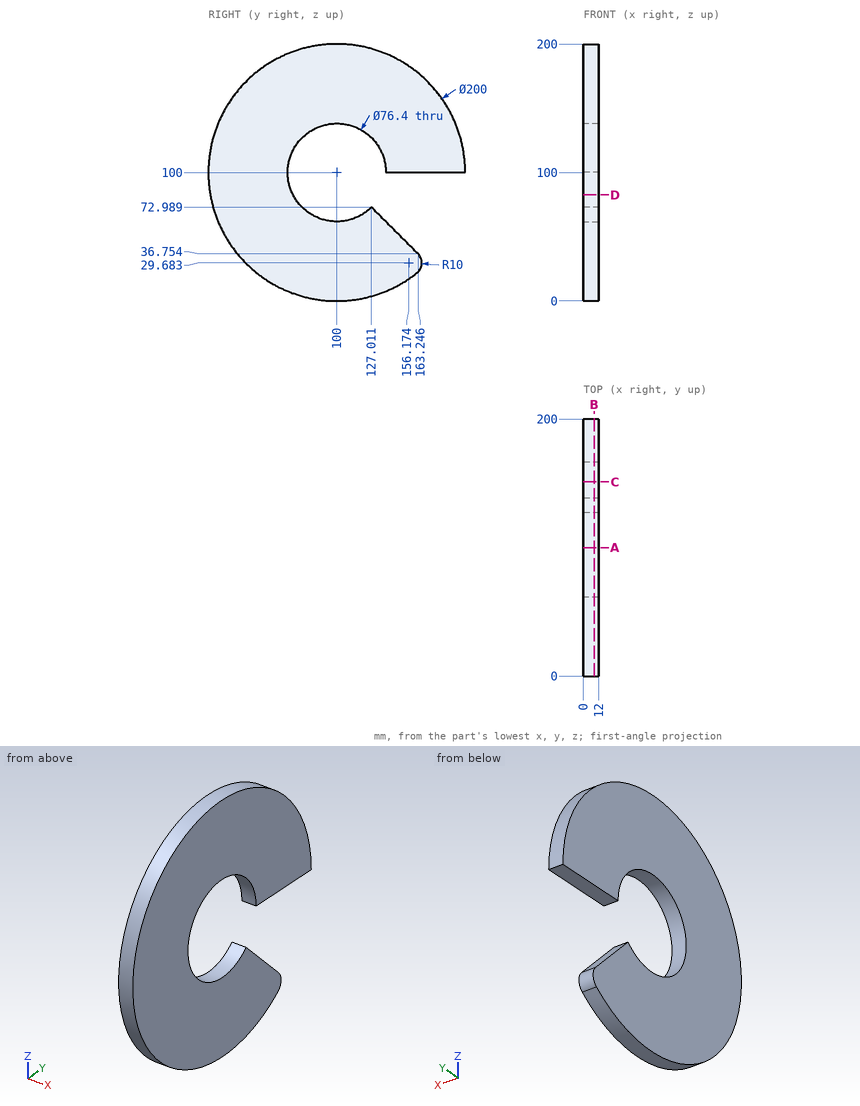
The drawing under review shows one solid part. Ordinate dimensions are in mm from its lowest x, y, z. Coordinates: 2 decimals unless noted, no trailing zeros. Loops run counter-clockwise (first coordinate to the right, second up) from the corner with the lowest first, then second, coordinate; pieces in that order, holes last. Notation, with made-up numbers: (72.5, 87.25) -> (76.5, 87.25) arc R24 ccw to (76.5, 119.25) -> close; hole circle Ø11 at (-20, -14.5). An arc over 180 degrees is marked (long way). Answer as a JSON object with one key per item and string values.
Q1. Take a section at C-C on y = 151. Give the boundary of the cut face in (x, z), plus the area to 3 significant figures.
Answer block:
{"outline": "(0, 13.98) -> (12, 13.98) -> (12, 49) -> (0, 49) -> close; (0, 100) -> (12, 100) -> (12, 186.02) -> (0, 186.02) -> close", "area": "1,450 mm^2"}
Q2. Clearance check with flat-ended pins moving along their axes: pin 1 Ø6 at (x, y) = (3.5, 171) entering from -Z; pin 2 Ø6 at (x, z) = (9, 78.5) entering from -Y; pin 3 Ø5 at (x, z) = (4, 145) entering from -Y. State where each tip first meets the part, or that it passes through.
Answer block:
{"pin 1": "stops at z = 100", "pin 2": "stops at y = 1.73", "pin 3": "stops at y = 9.48"}
Q3. Take a section at D-D on z = 82.5. Give the boundary of the cut face in (x, y) (1 decimal), plus the area to 3 significant figures.
Answer block:
{"outline": "(0, 1.5) -> (12, 1.5) -> (12, 66) -> (0, 66) -> close", "area": "774 mm^2"}
Q4. Take a section at A-A on y = 100. Give the boundary of the cut face in (x, z), plus the area to 3 significant figures.
Answer block:
{"outline": "(0, 0) -> (12, 0) -> (12, 61.8) -> (0, 61.8) -> close; (0, 138.2) -> (12, 138.2) -> (12, 200) -> (0, 200) -> close", "area": "1,480 mm^2"}
Q5. Take a section at B-B on x = 8.5. Give the boundary of the cut face in (y, z) (1 decimal).
Answer block:
{"outline": "(127, 73) arc R38.2 cw (long way) to (138.2, 100) -> (200, 100) arc R100 ccw (long way) to (162.4, 21.9) arc R10 ccw to (163.2, 36.8) -> close"}
Q6. To check wall thickness, follow L1, parallel to Z at x = 8, y = 100; L2, parallel to Z at x = 2.5, y = 175 (1 decimal); L3, parallel to Z at x = 3.25, y = 154 (1 decimal). State the ranges of each line that lie inside material, in increasing order.
Answer block:
{"L1": "z = 0 to 61.8, 138.2 to 200", "L2": "z = 100 to 166.1", "L3": "z = 15.8 to 46, 100 to 184.2"}
